Autodesk Inventor part; units mm, degrees
ref_plane "Plano de trabalho1" through (9.4, 0, 0) normal (1, 0, 0) x (0, 0, -1)
ref_plane "YZ Plane" through (0, 0, 0) normal (1, 0, 0) x (0, 1, 0)
ref_plane "XZ Plane" through (0, 0, 0) normal (0, 1, 0) x (-1, 0, 0)
sketch "Esboço1" plane through (0, 0, 0) normal (0, 0, 1) x (1, 0, 0)
  line L0 (0, 0) -> (18.8, 0)
  line L1 (18.8, 0) -> (18.8, 22.5)
  line L2 (18.8, 22.5) -> (0, 22.5)
  line L3 (0, 22.5) -> (0, 0)
  dimension "d0" = 18.8
  dimension "d1" = 22.5
extrude "Extrusão1" add sketch "Esboço1" along normal blind 64.2
sketch "Esboço2" plane through (18.8, 0, 0) normal (1, 0, 0) x (0, 0, -1)
  line L0 (0, 0) -> (-64.2, 0)
  line L1 (0, 0) -> (0, 11.25)
  line L2 (0, 0) -> (0, 22.5)
  line L3 (0, 11.25) -> (-11.2, 11.25)
  circle A0 centre (-11.2, 11.25) radius 2.7
  dimension "d4" = 11.25
  dimension "d5" = 11.2
  dimension "d6" = 5.4
extrude "Extrusão2" add sketch "Esboço2" along normal blind 1.1
sketch "Esboço3" plane through (19.9, 11.25, 11.2) normal (1, 0, 0) x (0, 0, -1)
  circle A0 centre (0, 0) radius 1.8
  point P0 (11.2, -11.25)
  dimension "d9" = 3.6
extrude "Extrusão3" add sketch "Esboço3" along normal blind 7.9
ref_plane "Plano de trabalho1" through (9.4, 0, 0) normal (1, 0, 0) x (0, 0, -1)
mirror "Espelhamento1" about plane through (9.4, 0, 0) normal (1, 0, 0) of "Extrusão3", "Extrusão2"
fillet "Arredondamento1" radius 2 1 edges at (9.4, 22.5, 0)
fillet "Arredondamento2" radius 2 1 edges at (9.4, 0, 0)
sketch "Esboço4" plane through (18.8, 0, 64.2) normal (1, 0, 0) x (0, 0, -1)
  line L0 (64.2, 0) -> (32.4, 0)
  line L1 (62.2, 0) -> (0, 0)
  line L2 (32.4, 0) -> (32.4, 2.5)
  circle A0 centre (32.4, 2.5) radius 1.5
  line L3 (32.4, 2.5) -> (32.4, 20)
  circle A1 centre (32.4, 20) radius 1.5
  dimension "d15" = 31.8
  dimension "d16" = 2.5
  dimension "d17" = 3
  dimension "d18" = 17.5
  dimension "d19" = 3
extrude "Extrusão4" cut sketch "Esboço4" against normal through all
sketch "Esboço5" plane through (0, 0, 64.2) normal (0, 0, 1) x (1, 0, 0)
  line L0 (18.8, 22.5) -> (0, 22.5)
  line L1 (0, 22.5) -> (18.8, 22.5)
  line L2 (18.8, 22.5) -> (18.8, 0)
  line L3 (18.8, 0) -> (0, 0)
  line L4 (0, 0) -> (0, 22.5)
  arc A0 (18.8, 17.831338) -> (0, 17.831338) centre (9.4, 10.702573) ccw
  point P0 (9.4, 22.5)
extrude "Extrusão5" cut sketch "Esboço5" against normal blind 23.8 contours L2 A0 L0 | A0 L4 L0
sketch "Esboço6" plane through (0, 0, 64.2) normal (0, 0, 1) x (1, 0, 0)
  line L0 (0, 22.508504) -> (18.8, 22.508504)
  line L1 (18.8, 22.508504) -> (18.8, 0)
  line L2 (18.8, 0) -> (0, 0)
  line L3 (0, 0) -> (0, 22.508504)
  arc A0 (0, 6.267075) -> (18.8, 6.372369) centre (9.378542, 10.150894) ccw
  point P0 (9.357085, 0)
  point P1 (9.4, 0)
extrude "Extrusão6" cut sketch "Esboço6" against normal blind 23.8 contours A0 L2 L3 | L1 L2 A0
sketch "Esboço7" plane through (0, 0, 64.2) normal (0, 0, 1) x (1, 0, 0)
  line L0 (0, 22.5) -> (9.4, 22.5)
  line L1 (0, 22.5) -> (18.8, 22.5)
  line L2 (18.8, 22.5) -> (18.8, 0)
  line L3 (18.8, 0) -> (0, 0)
  line L4 (0, 0) -> (0, 22.5)
  arc A0 (18.8, 14.455208) -> (0, 14.564328) centre (9.378542, 10.812909) ccw
extrude "Extrusão7" cut sketch "Esboço7" against normal blind 11.9 contours L0 L1 L2 A0 L4
sketch "Esboço9" plane through (0, 0, 64.2) normal (0, 0, 1) x (1, 0, 0)
  line L0 (0, 20.5) -> (0, 2)
  line L1 (18.8, 13.95) -> (18.8, 8.55)
  arc A0 (0, 11.25) -> (18.8, 11.25) centre (9.4, 10.967634) ccw
  line L2 (0, 20.5) -> (0, 22.5)
  line L3 (0, 22.5) -> (18.8, 22.5)
  line L4 (18.8, 22.5) -> (18.8, 0)
  line L5 (18.8, 0) -> (0, 0)
  line L6 (0, 0) -> (0, 22.5)
  point P0 (18.8, 10.685268)
  point P1 (0, 10.685268)
sketch "Esboço9 outline for Extrusão8" plane through (0, 0, 64.2) normal (0, 0, 1) x (1, 0, 0)
  line L0 (0, 0) -> (18.8, 0)
  line L1 (0, 2) -> (0, 0)
  line L2 (0, 10.685268) -> (0, 2)
  arc A0 (18.8, 10.685268) -> (0, 10.685268) centre (9.4, 10.967634) cw
  line L3 (18.8, 8.55) -> (18.8, 10.685268)
  line L4 (18.8, 0) -> (18.8, 8.55)
extrude "Extrusão8" cut sketch "Esboço9 outline for Extrusão8" against normal blind 11.9
properties part number "motorDC"
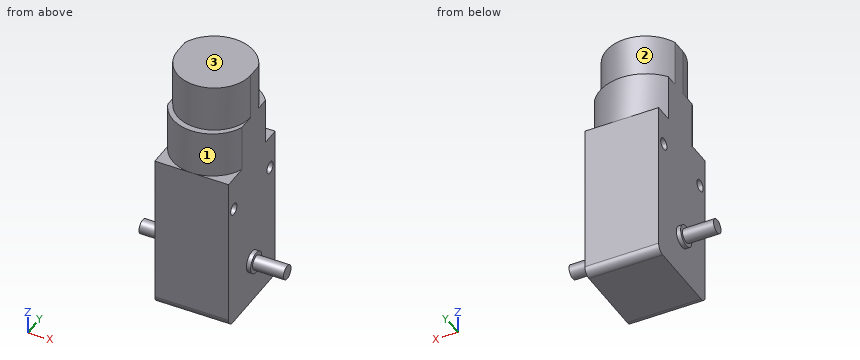
Verification items for the finished model (mm, model axes). Face numbers are marked on the shaded views. A direction names the side the tool comes from. Round coordinates to 2 decimals unless told otherwise and drop trailing zeros. Loops run counter-clockwise (first coordinate to the right, second up) from the corner with the lowest first, then second, coordinate; pieces in that order, holes last. Notation, with made-up numbers: (0.25, 33.5) -> (16.25, 33.5) arc R36 cw to (16.25, 71.5) -> close; hole circle Ø7 at (13.5, -24). An arc over 180 degrees is marked (long way). Answer as a JSON object with one key per item and string values.
Q1. Go/stop test with flat-tipped pins: P1, Ø5, axis at y = 14, z = 30, coming from the +X side; P2, Ø10, axis at x = 24, y = 13, coming from the -Z side; P3, Ø6, axis at x = 23, y = 15.5, coming from the +Z side. Record where each tip stops, or that it passes through.
Data:
{"P1": "stops at x = 18.8", "P2": "stops at z = 8.5", "P3": "stops at z = 12.5"}
Q2. Section check C-C (z = 11.2). Record the boundary of the cut face in (x, y), then the cut area to 3 significant figures.
Data:
{"outline": "(-9, 9.45) -> (-1.1, 9.45) -> (-1.1, 8.55) -> (0, 8.55) -> (0, 0) -> (18.8, 0) -> (18.8, 8.55) -> (19.9, 8.55) -> (19.9, 9.45) -> (27.8, 9.45) -> (27.8, 13.05) -> (19.9, 13.05) -> (19.9, 13.95) -> (18.8, 13.95) -> (18.8, 22.5) -> (0, 22.5) -> (0, 13.95) -> (-1.1, 13.95) -> (-1.1, 13.05) -> (-9, 13.05) -> close", "area": "492 mm2"}
Q3. Section check B-B (x = 4.5). Record the boundary of the cut face in (y, z), then the cut area to 3 significant figures.
Data:
{"outline": "(0, 2) arc R2 ccw to (2, 0) -> (20.5, 0) arc R2 ccw to (22.5, 2) -> (22.5, 40.4) -> (21.43, 40.4) -> (21.43, 52.3) -> (19.66, 52.3) -> (19.66, 64.2) -> (2.94, 64.2) -> (2.94, 52.3) -> (1.25, 52.3) -> (1.25, 40.4) -> (0, 40.4) -> close; hole circle Ø3 at (2.5, 31.8); hole circle Ø3 at (20, 31.8)", "area": "1,330 mm2"}
Q4. Section check A-A (z = 31.8). Record the boundary of the cut face in (x, y).
Data:
{"outline": "(0, 0) -> (18.8, 0) -> (18.8, 1) -> (0, 1) -> close; (0, 4) -> (18.8, 4) -> (18.8, 18.5) -> (0, 18.5) -> close; (0, 21.5) -> (18.8, 21.5) -> (18.8, 22.5) -> (0, 22.5) -> close"}
Q5. Access from +Z, -Z, +X, -X, +Y, -Y to the whole of each face (thin tool, end or side, straight path). Record for the marked faces 1, 2 and 3.
Data:
{"face 1": "+Z, -Y", "face 2": "+Z, +Y", "face 3": "+Z, +X, -X, +Y, -Y"}
Q6. Section check D-D (x = -2). Record the boundary of the cut face in (y, z).
Data:
{"outline": "circle Ø3.6 at (11.25, 11.2)"}
Q7. Scan lines: line 1 (Y direction, x = 9.25, z = 31.8); line 2 (Z direction, x = 15, y = 2.5); line 3 (Z direction, x = 11.5, y = 2.5). Record each from-to range of solid material in increasing order. Write a range as from..to.
Data:
{"line 1": "y = 0..1, 4..18.5, 21.5..22.5", "line 2": "z = 0..30.3, 33.3..52.3", "line 3": "z = 0..30.3, 33.3..64.2"}
